Read the model definition and answer for the solid it produces. Units are mm, in the model's axes. A direction names the side the tool comes from. Give positions to 0.01 mm unless a question says otherwise; leave off trailing zeros. Order: outer loops, then holes, each group sorted by start corner. A loop starts at its lowest first (then second) coordinate and runs counter-clockwise, first axis right, second up. Notation, with made-up numbers: (-34.75, 82.25) - (14.25, 82.25) arc R10 ccw to (14.25, 97.25) - close; hole circle Ø10 at (62.5, 3). An arc over 180 degrees is marked (long way). Use a Markdown table: item, result. Add a question column.
1. For a pull along Z with two mould halves and no side action, classify faces 5 (the flat face through (-10.75, -3, 12)), 6 (the flat face through (-13, -9, 0)), 7 (the cylindrical face through (16.428, -28.771, 11.765)) as released by +Z, released by -Z, zero draft, split by the parting line, or undercut.
2. Flat-ended cylindrical pins translate along their axes: P1, Ø2, axis at x = 11.5, z = 8.5, coming from the +Y side; P2, Ø12, axis at y = -12.5, z = 9, coming from the -X side; P3, Ø6, axis at y = 0, z = 23.5, coming from the +X side. Find the tip coordinate at first contact, or state that the pin passes through.
3. Consider L1, parallel to X at y = -20.5, z = 2.25; L2, parallel to Z at x = 16, y = -29; L3, parallel to Z at x = 1.5, y = -8.5. Determine where each line is inside the solid, lowest interval first.
4. A cutting plane is placed at D-D on x = -16.2. Determine the outline of the cut face in (y, z).
5. A cutting plane is placed at C-C on z = 10.5. Determine the outline of the cut face in (x, y), and give its area (3 significant figures).
6. Which of the six approach directions +Z, -Z, +X, -X, +Y, -Y give full straight-line access (tool end or side, diameter ignored) to faces 1 (the cylindrical face through (-3.25, 25.67, 22)), 2 (the flat face through (-1.15, 25.3, 8.6)), 3 (the cylindrical face through (11.99, 21.75, 22.57)), 4 (the flat face through (-14, -27.25, 13))?
7. A cutting plane is placed at A-A on z = 3. Determine the outline of the cut face in (x, y).
8. A cutting plane is placed at B-B on x = 0. Determine the outline of the cut face in (y, z).
```python
from build123d import *

# Parameters (mm, degrees)
SKETCH_1_W          = 26.4
SKETCH_1_H          = 60.5
EXTRUDE_1_DEPTH     = 27
SKETCH_3_W          = 21.5
SKETCH_3_H          = 60.5
CUT_EXTRUDE_1_DEPTH = 24
SKETCH_4_W          = 24
SKETCH_4_H          = 10
CUT_EXTRUDE_2_DEPTH = 27.4
SKETCH_7_W          = 2.3
SKETCH_7_H          = 8
EXTRUDE_3_DEPTH     = 24
CUT_EXTRUDE_4_REACH = 16.35
SKETCH_9_R          = 1.75
FILLET_1_R          = 7
FILLET_2_R          = 7
FILLET_3_R          = 4
FILLET_4_R          = 0.2
FILLET_7_R          = 5
SKETCH_10_R         = 1
CUT_EXTRUDE_5_DEPTH = 61.5000001
SKETCH_11_W         = 6
SKETCH_11_H         = 27
SKETCH_11_R         = 1.75
EXTRUDE_4_DEPTH     = 3


with BuildPart() as part:
    # ｽｹｯﾁ1 → ﾎﾞｽ - 押し出し1 (new body)
    with BuildSketch(Plane.XY):
        Rectangle(SKETCH_1_W, SKETCH_1_H)
    extrude(amount=EXTRUDE_1_DEPTH)

    # ｽｹｯﾁ3 → ｶｯﾄ - 押し出し1 (cut)
    with BuildSketch(Plane(origin=(0, 0, 0), x_dir=(-1, 0, 0), z_dir=(0, 0, -1))):
        Rectangle(SKETCH_3_W, SKETCH_3_H)
    extrude(amount=-CUT_EXTRUDE_1_DEPTH, mode=Mode.SUBTRACT)

    # ｽｹｯﾁ4 → ｶｯﾄ - 押し出し2 (cut, through all)
    with BuildSketch(Plane.ZY.offset(13.2)):
        with Locations((12, 25.25)):
            Rectangle(SKETCH_4_W, SKETCH_4_H)
    extrude(amount=-CUT_EXTRUDE_2_DEPTH, mode=Mode.SUBTRACT)

    # ｽｹｯﾁ7 → ﾎﾞｽ - 押し出し3 (add)
    with BuildSketch(Plane(origin=(0, 0, 24), x_dir=(-1, 0, 0), z_dir=(0, 0, -1))):
        with Locations((0, 26.25)):
            Rectangle(SKETCH_7_W, SKETCH_7_H)
    extrude(amount=EXTRUDE_3_DEPTH)

    # ｽｹｯﾁ9 → ｶｯﾄ - 押し出し4 (cut, up to next)
    with BuildSketch(Plane(origin=(1.15, 0, 0), x_dir=(0, 0, -1), z_dir=(1, 0, 0)), mode=Mode.PRIVATE) as cut_extrude_4_sk1:
        with Locations((-10.5, 26.25)):
            Circle(SKETCH_9_R)
    cut_extrude_4_tool1 = extrude(cut_extrude_4_sk1.sketch, amount=-CUT_EXTRUDE_4_REACH, mode=Mode.PRIVATE) & part.part
    add(cut_extrude_4_tool1.solids().sort_by_distance((1.15, 26.25, 10.5))[0], mode=Mode.SUBTRACT)

    # ﾌｨﾚｯﾄ1
    fillet_1_edges = [part.edges().sort_by_distance(p)[0] for p in [
        (1.15, 26.25, 24),
    ]]
    fillet(fillet_1_edges, radius=FILLET_1_R)

    # ﾌｨﾚｯﾄ2
    fillet_2_edges = [part.edges().sort_by_distance(p)[0] for p in [
        (-1.15, 26.25, 24),
    ]]
    fillet(fillet_2_edges, radius=FILLET_2_R)

    # ﾌｨﾚｯﾄ3
    fillet_3_edges = [part.edges().sort_by_distance(p)[0] for p in [
        (0, 22.25, 24),
    ]]
    fillet(fillet_3_edges, radius=FILLET_3_R)

    # ﾌｨﾚｯﾄ4
    fillet_4_edges = [part.edges().sort_by_distance(p)[0] for p in [
        (1.15, 26.25, 12.25),
        (-1.15, 26.25, 12.25),
    ]]
    fillet(fillet_4_edges, radius=FILLET_4_R)

    # ﾌｨﾚｯﾄ7
    fillet_7_edges = [part.edges().sort_by_distance(p)[0] for p in [
        (11.975, 20.25, 24),
        (-11.975, 20.25, 24),
    ]]
    fillet(fillet_7_edges, radius=FILLET_7_R)

    # ｽｹｯﾁ10 → ｶｯﾄ - 押し出し5 (cut, through all)
    with BuildSketch(Plane(origin=(0, -30.25, 0), x_dir=(-1, 0, 0), z_dir=(0, -1, 0))):
        with Locations((0, -27)):
            Circle(SKETCH_10_R)
    extrude(amount=-CUT_EXTRUDE_5_DEPTH, mode=Mode.SUBTRACT)

    # ｽｹｯﾁ11 → ﾎﾞｽ - 押し出し4 (add)
    with BuildSketch(Plane(origin=(0, -30.25, 0), x_dir=(-1, 0, 0), z_dir=(0, -1, 0))):
        with Locations((-16.2, -13.5)):
            Rectangle(SKETCH_11_W, SKETCH_11_H)
        with Locations((-16.2, -13.5)):
            Circle(SKETCH_11_R, mode=Mode.SUBTRACT)
        with Locations((16.2, -13.5)):
            Rectangle(SKETCH_11_W, SKETCH_11_H)
        with Locations((16.2, -13.5)):
            Circle(SKETCH_11_R, mode=Mode.SUBTRACT)
    extrude(amount=-EXTRUDE_4_DEPTH)


solid = part.part
```
Output values:
| question | item | result |
|---|---|---|
| 1 | face 5 | zero draft |
| 1 | face 6 | released by -Z |
| 1 | face 7 | undercut |
| 2 | P1 | y = 20.25 |
| 2 | P2 | x = -13.2 |
| 2 | P3 | x = 13.2 |
| 3 | L1 | -13.2 to -10.75, 10.75 to 13.2 |
| 3 | L2 | 0 to 11.76, 15.24 to 27 |
| 3 | L3 | 24 to 27 |
| 4 | outline | (-30.25, 0) - (-27.25, 0) - (-27.25, 11.75) - (-30.25, 11.75) - close; (-30.25, 15.25) - (-27.25, 15.25) - (-27.25, 27) - (-30.25, 27) - close |
| 5 | outline | (-19.2, -30.25) - (-10.75, -30.25) - (-10.75, 20.25) - (-13.2, 20.25) - (-13.2, -27.25) - (-19.2, -27.25) - close; (-1.15, 22.25) - (1.15, 22.25) - (1.15, 24.3) arc R0.2 ccw to (0.95, 24.5) - (-0.95, 24.5) arc R0.2 ccw to (-1.15, 24.3) - close; (-1.15, 28.2) arc R0.2 ccw to (-0.95, 28) - (0.95, 28) arc R0.2 ccw to (1.15, 28.2) - (1.15, 30.25) - (-1.15, 30.25) - close; (10.75, -30.25) - (19.2, -30.25) - (19.2, -27.25) - (13.2, -27.25) - (13.2, 20.25) - (10.75, 20.25) - close |
| 5 | area | 294 mm² |
| 6 | face 1 | -Z, +Y, -Y |
| 6 | face 2 | -Z, -X, +Y, -Y |
| 6 | face 3 | -Z, +X, +Y |
| 6 | face 4 | +Z, -Z, -X, +Y |
| 7 | outline | (-19.2, -30.25) - (-10.75, -30.25) - (-10.75, 20.25) - (-13.2, 20.25) - (-13.2, -27.25) - (-19.2, -27.25) - close; (-1.15, 22.25) - (1.15, 22.25) - (1.15, 30.25) - (-1.15, 30.25) - close; (10.75, -30.25) - (19.2, -30.25) - (19.2, -27.25) - (13.2, -27.25) - (13.2, 20.25) - (10.75, 20.25) - close |
| 8 | outline | (-30.25, 24) - (18.25, 24) arc R4 cw to (22.25, 20) - (22.25, 0) - (30.25, 0) - (30.25, 26) - (-30.25, 26) - close; hole circle Ø3.5 at (26.25, 10.5) |
